```python
from build123d import *

# Parameters (mm, degrees)
SKETCH1_R           = 1.9
BOSS_EXTRUDE1_DEPTH = 55
SKETCH2_W           = 17
SKETCH2_H           = 8
BOSS_EXTRUDE2_DEPTH = 3
SKETCH3_R           = 1.5
CUT_EXTRUDE1_DEPTH  = 53.841744861
SKETCH4_W           = 5
SKETCH4_H           = 8
BOSS_EXTRUDE3_DEPTH = 40


with BuildPart() as part:
    # Sketch1 → Boss-Extrude1 (new body)
    with BuildSketch(Plane(origin=(0, 0, 0), x_dir=(1, 0, 0), z_dir=(0, 1, 0))):
        with Locations(Location((0, 0, 0), (0, 0, 270))):
            Circle(SKETCH1_R)
    extrude(amount=BOSS_EXTRUDE1_DEPTH)

    # Sketch2 → Boss-Extrude2 (add)
    with BuildSketch(Plane.XZ):
        Rectangle(SKETCH2_W, SKETCH2_H)
    extrude(amount=-BOSS_EXTRUDE2_DEPTH)

    # Sketch3 → Cut-Extrude1 (cut, through all)
    with BuildSketch(Plane(origin=(0, 3, 0), x_dir=(1, 0, 0), z_dir=(0, 1, 0))):
        with Locations(Location((-5.5, 0, 0), (0, 0, 270))):
            Circle(SKETCH3_R)
        with Locations(Location((5.5, 0, 0), (0, 0, 90))):
            Circle(SKETCH3_R)
    extrude(amount=-CUT_EXTRUDE1_DEPTH, mode=Mode.SUBTRACT)

    # Sketch4 → Boss-Extrude3 (add)
    with BuildSketch(Plane(origin=(0, 3, 0), x_dir=(1, 0, 0), z_dir=(0, 1, 0))):
        Rectangle(SKETCH4_W, SKETCH4_H)
    extrude(amount=BOSS_EXTRUDE3_DEPTH)


solid = part.part
```
Geometry: final body of the model. Coordinates: model frame, mm. A direction names the side the tool comes from. Round coordinates to 2 decimals unless told otherwise and drop trailing zeros. Order: outer loops, then holes, each group sorted by start corner. A loop starts at its lowest first (then second) coordinate and runs counter-clockwise, first axis right, second up. Notation, with made-up numbers: M -34,-21.75 L -28,-21.75 A23 cw -28,15.25 Z; hole C -25.75,-17.75 d6. An arc over 180 degrees is marked long. One line per item, written item: value.
(1) Cut plane B-B (z = -2.5). Return the cut outline in (x, y), and give its area (3 significant figures).
Result sheet:
outline: M -8.5,0 L 8.5,0 L 8.5,3 L 2.5,3 L 2.5,43 L -2.5,43 L -2.5,3 L -8.5,3 Z
area: 251 mm2
(2) Line query: probe 1 along X at (y, z) = (2.3, 0); probe 2 along Z at (x, y) = (5.5, 2.25); probe 3 along X at (y, z) = (22.5, 2.5). Output: solid intervals per line, ascending. Write a range as [from, to].
Result sheet:
probe 1: [-8.5, -7], [-4, 4], [7, 8.5]
probe 2: [-4, -1.5], [1.5, 4]
probe 3: [-2.5, 2.5]
(3) Pin query (flat end, axial travel): P1, Ø3, axis at x = 5, z = 2, coming from the +Y side; P2, Ø1.5, axis at y = 10, z = -1.5, coming from the +X side; P3, Ø4, axis at x = -3.5, z = 3, coming from the +Y side. Return the tip coordinate at first contact, or that it passes through.
Result sheet:
P1: y = 3
P2: x = 2.5
P3: y = 43
(4) Cut plane C-C (z = 0). Return the cut outline in (x, y).
Result sheet:
outline: M -8.5,0 L -7,0 L -7,3 L -8.5,3 Z; M -4,0 L 4,0 L 4,3 L 2.5,3 L 2.5,43 L 1.9,43 L 1.9,55 L -1.9,55 L -1.9,43 L -2.5,43 L -2.5,3 L -4,3 Z; M 7,0 L 8.5,0 L 8.5,3 L 7,3 Z
(5) Cut plane A-A (x = -5.5). Return the cut outline in (y, z).
Result sheet:
outline: M 0,-4 L 3,-4 L 3,-1.5 L 0,-1.5 Z; M 0,1.5 L 3,1.5 L 3,4 L 0,4 Z
(6) Cut plane D-D (x = 0). Return the cut outline in (y, z).
Result sheet:
outline: M 0,-4 L 43,-4 L 43,-1.9 L 55,-1.9 L 55,1.9 L 43,1.9 L 43,4 L 0,4 Z
(7) Reachability of faces 1 (the flat face through (-1, 43, -2)), 2 (the flat face through (-4, 3, 1)), 3 (the flat face through (2.5, 23, 0)), 4 (the flat face through (0, 55, 0)) from +Z, -Z, +X, -X, +Y, -Y: full face, straight path, thin tool, end or side. Return the list, or none.
Result sheet:
face 1: +Y
face 2: +Z, -Z, -X, +Y
face 3: +Z, -Z, +X, +Y
face 4: +Z, -Z, +X, -X, +Y
